```python
from build123d import *

# Parameters (mm, degrees)
SKETCH1_W           = 10
SKETCH1_H           = 3
BOSS_EXTRUDE1_DEPTH = 3


with BuildPart() as part:
    # Sketch1 → Boss-Extrude1 (new body)
    with BuildSketch(Plane.XY):
        Polygon((21, -78.90992989), (-21, -78.90992989), (-21, 29.09007011), (-5, 29.09007011), (21, 29.09007011), align=None)
        with BuildLine():
            Line((-13.5, -38.90992989), (-13.5, -68.90992989))
            ThreePointArc((-13.5, -68.90992989), (-16, -71.40992989), (-18.5, -68.90992989))
            Line((-18.5, -68.90992989), (-18.5, -38.90992989))
            ThreePointArc((-18.5, -38.90992989), (-16, -36.40992989), (-13.5, -38.90992989))
        make_face(mode=Mode.SUBTRACT)
        with BuildLine():
            Line((18.5, -38.90992989), (18.5, -68.90992989))
            ThreePointArc((18.5, -68.90992989), (16, -71.40992989), (13.5, -68.90992989))
            Line((13.5, -68.90992989), (13.5, -38.90992989))
            ThreePointArc((13.5, -38.90992989), (16, -36.40992989), (18.5, -38.90992989))
        make_face(mode=Mode.SUBTRACT)
        with Locations((0, 22.59007011)):
            Rectangle(SKETCH1_W, SKETCH1_H, mode=Mode.SUBTRACT)
    extrude(amount=BOSS_EXTRUDE1_DEPTH)


solid = part.part
```
Here's how the part is built. I have some questions about the finished solid (model axes, mm). A direction names the side the tool comes from. Give positions to 0.01 mm unless a question says otherwise; leave off trailing zeros. Write each loop counter-clockwise with the first axis right and the second up, starting at its lowest first coordinate (ties: lowest second). Pieces come first, ordered by that corner, then holes. Notation, with made-up numbers: (7.5, 42.25) -> (43.5, 42.25) arc R17 ccw to (43.5, 47.25) -> close; hole circle Ø4 at (58.5, -18). An arc over 180 degrees is marked (long way). Use one line per item in the form item = value.
1) Suppose I cut it at A-A (y = -42.5). Please give me the cut outline in (x, z), and give its area (3 significant figures).
Verdict:
outline = (-21, 0) -> (-18.5, 0) -> (-18.5, 3) -> (-21, 3) -> close; (-13.5, 0) -> (13.5, 0) -> (13.5, 3) -> (-13.5, 3) -> close; (18.5, 0) -> (21, 0) -> (21, 3) -> (18.5, 3) -> close
area = 96.0 mm2
2) On a 3-axis mill with a long thin cutter (end or side, diameter ignored), from which of +Z, -Z, +X, -X, +Y, -Y can I reach the whole of each face in a straight line? I mean faces 4 (the face through (-18.5, -54, 1)), 5 (the face through (21, -24, 1)). Say none if no direction works.
Verdict:
face_4 = +Z, -Z
face_5 = +Z, -Z, +X, +Y, -Y
3) Suppose I cut it at C-C (z = 1.9). Please give me the cut outline in (x, y), and give its area (3 significant figures).
Verdict:
outline = (-21, -78.91) -> (21, -78.91) -> (21, 29.09) -> (-21, 29.09) -> close; hole (-18.5, -68.91) arc R2.5 ccw to (-13.5, -68.91) -> (-13.5, -38.91) arc R2.5 ccw to (-18.5, -38.91) -> close; hole (-5, 21.09) -> (5, 21.09) -> (5, 24.09) -> (-5, 24.09) -> close; hole (13.5, -68.91) arc R2.5 ccw to (18.5, -68.91) -> (18.5, -38.91) arc R2.5 ccw to (13.5, -38.91) -> close
area = 4,170 mm2
4) Suppose I cut it at B-B (x = -4). Please give me the cut outline in (y, z), and give its area (3 significant figures).
Verdict:
outline = (-78.91, 0) -> (21.09, 0) -> (21.09, 3) -> (-78.91, 3) -> close; (24.09, 0) -> (29.09, 0) -> (29.09, 3) -> (24.09, 3) -> close
area = 315 mm2
5) We'd pull the mould along X, two halves only. Please class faces 1 (the face through (16.05, -71.41, 1.48)), 2 (the face through (0, -24, 3)), 3 (the face through (-21, -26, 1)): +X half, -X half, draft (parallel to the pull), parting line (faces both ways), or undercut.
Verdict:
face_1 = undercut
face_2 = draft
face_3 = -X half
6) If I drill on L1, parallel to X at y = -40, z = 1.4; L2, parallel to Y at x = -3, z = 2.45; L3, parallel to X at y = 22, z = 1.95, over which ranges is the centre line in solid material (lowest first)? Write a range as [from, to].
Verdict:
L1 = [-21, -18.5], [-13.5, 13.5], [18.5, 21]
L2 = [-78.91, 21.09], [24.09, 29.09]
L3 = [-21, -5], [5, 21]
7) Suppose I cut it at D-D (x = -16). Please give me the cut outline in (y, z), and give its area (3 significant figures).
Verdict:
outline = (-78.91, 0) -> (-71.41, 0) -> (-71.41, 3) -> (-78.91, 3) -> close; (-36.41, 0) -> (29.09, 0) -> (29.09, 3) -> (-36.41, 3) -> close
area = 219 mm2
